Read the model definition and answer for the solid it produces. Units are mm, in the model's axes. Face numbers are marked on the shaded views. A direction names the side the tool comes from. Give positions to 0.01 mm unless a question says otherwise; leave off trailing zeros. Write each loop counter-clockwise with the first axis right and the second up, starting at its lowest first coordinate (ties: lowest second). Pieces come first, ordered by that corner, then holes. Notation, with made-up numbers: (12.25, 62) -> (27.25, 62) arc R22 cw to (27.25, 69) -> close; hole circle Ø11 at (-3, 57). An arc over 180 degrees is marked (long way). Put each result on its own line as item: value. Start each with the question number.
from build123d import *

# Parameters (mm, degrees)
F0_W     = 23.5
F0_H     = 8
F1_DEPTH = 4.1
F2_W     = 4.6
F2_H     = 8
F3_DEPTH = 5
F4_SIZE  = 5


with BuildPart() as f1:
    # F0 (on Top) → F1 (new body)
    with BuildSketch(Plane.XY):
        Rectangle(F0_W, F0_H)
    extrude(amount=F1_DEPTH)

    # F2 (on face) → F3 (join)
    with BuildSketch(Plane.XY.offset(4.1)):
        with Locations((-9.45, 0)):
            Rectangle(F2_W, F2_H)
        with Locations((9.45, 0)):
            Rectangle(F2_W, F2_H)
    extrude(amount=F3_DEPTH)

    # F4
    f4_edges = [f1.edges().sort_by_distance(p)[0] for p in [
        (-9.45, -4, 9.1),
        (9.45, -4, 9.1),
    ]]
    chamfer(f4_edges, length=F4_SIZE)


solid = f1.part
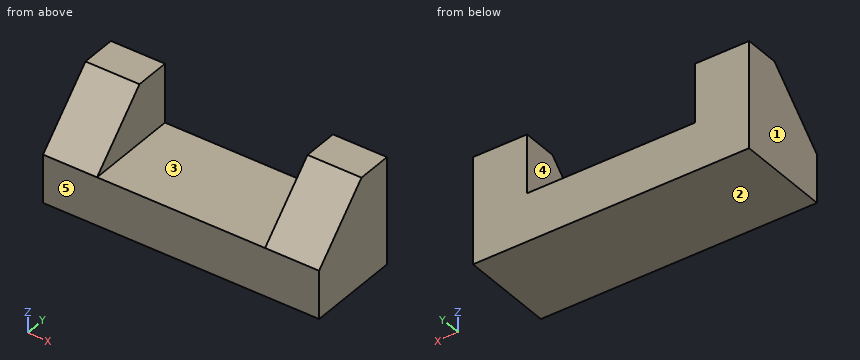
1) Straight lines are drawn through the part: line 1 (X direction, y = -1.75, z = 6); line 2 (Z direction, x = 3.25, y = 1.5); line 3 (Z direction, x = 7.75, y = 0). For each, find the intervals that lie inside material, in ascending order. Write a range as [from, to].
2) This flat-tipped pin is pushed along its axis until it touches: pin 1 Ø3 at (x, y) = (0, -2.5) entering from +Z. Where does it stop, or does it pass through?
3) A cutting plane is placed at C-C on z = 5.25. Give the vertices of the cut face in (x, y), and give its area (3 significant figures).
4) A cutting plane is placed at B-B on y = 2. Give the vertices of the cut face in (x, z).
5) A cutting plane is placed at A-A on z = 8.5. Give the vertices of the cut face in (x, y), and give its area (3 significant figures).
6) For a pull along X with two mould halves and no side action, classify the marked faces 1, 2 and 3 as pulls with the +X half, pulls with the -X half, needs draft (parallel to the pull), parting line crosses it, or undercut.
7) A cutting plane is placed at D-D on x = -10. Give the vertices of the cut face in (y, z).
8) For the marked faces 4 and 5, determine the directions among +Z, -Z, +X, -X, +Y, -Y from which every point of the face is accessible in a straight line to the end or side of a thin tool.
Results found:
1. line 1: x = [-11.75, -7.15], [7.15, 11.75]
1. line 2: z = [0, 4.1]
1. line 3: z = [0, 8.1]
2. pin 1: stops at z = 4.1
3. outline: (-11.75, -2.85) -> (-7.15, -2.85) -> (-7.15, 4) -> (-11.75, 4) -> close; (7.15, -2.85) -> (11.75, -2.85) -> (11.75, 4) -> (7.15, 4) -> close
3. area: 63.0 mm²
4. outline: (-11.75, 0) -> (11.75, 0) -> (11.75, 9.1) -> (7.15, 9.1) -> (7.15, 4.1) -> (-7.15, 4.1) -> (-7.15, 9.1) -> (-11.75, 9.1) -> close
5. outline: (-11.75, 0.4) -> (-7.15, 0.4) -> (-7.15, 4) -> (-11.75, 4) -> close; (7.15, 0.4) -> (11.75, 0.4) -> (11.75, 4) -> (7.15, 4) -> close
5. area: 33.1 mm²
6. face 1: pulls with the -X half
6. face 2: needs draft
6. face 3: undercut
7. outline: (-4, 0) -> (4, 0) -> (4, 9.1) -> (1, 9.1) -> (-4, 4.1) -> close
8. face 4: +Z, +Y, -Y
8. face 5: +Z, -Z, +X, -X, -Y
